Could you check a few things on this drawing? It's one solid part, dimensions in mm from its lowest x, y, z. A direction names the side the tool comes from. Round coordinates to 2 decimals unless told otherwise and drop trailing zeros. Loops run counter-clockwise (first coordinate to the right, second up) from the corner with the lowest first, then second, coordinate; pieces in that order, holes last. Notation, with made-up numbers: M 70.5,62 L 123.5,62 A21 ccw 123.5,91 Z; hole C -6.5,83.5 d1. An arc over 180 degrees is marked long. Put each result on its own line as item: value. Start each with the question number.
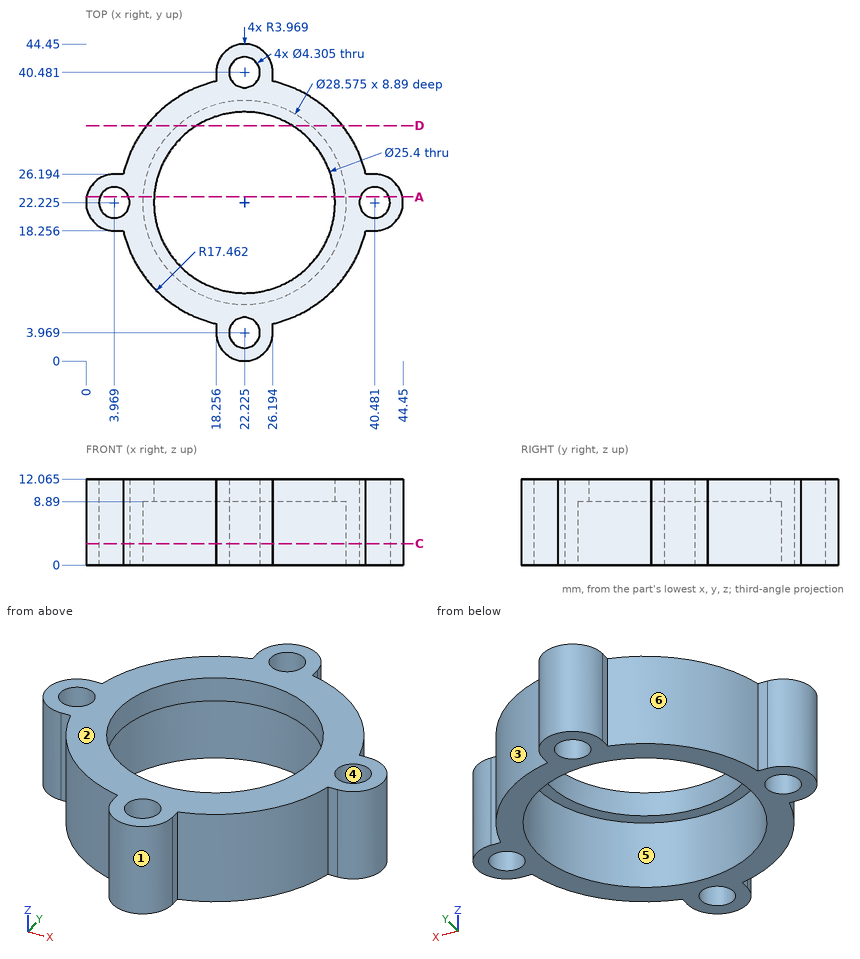
1) If we mould it in two halves opening along Y, with no side actions, what happens to the marked faces 1, 2, 3 and 4? For each: pulls with the +Y half, pulls with the -Y half, needs draft (parallel to the pull), parting line crosses it, or undercut.
2) Suppose I cut it at A-A (y = 23). Write out the boundary of the cut face in (x, z) (1 decimal), plus the area to 3 significant figures.
3) Suppose I cut it at C-C (z = 3). Write out the boundary of the cut face in (x, y) (1 decimal).
4) I'm going to push flat-ended pins straight in: P1, Ø0.6, axis at y = 40, z = 5, coming from the +X side; P2, Ø1, axis at x = 40, z = 8.5, coming from the +Y side; P3, Ø6, axis at y = 12, z = 8, coming from the -X side; P4, Ø8.5, axis at x = 18.5, y = 17.5, coming from the -Z side. Where does each tip first touch, or does it pass through?
5) If I drill on probe 1 along X at (y, z) = (40.5, 10); probe 2 along X at (y, z) = (34, 7) (1 decimal), over which ranges is the centre line in solid material (lowest first)? Write a range as from..to.
6) On a 3-axis mill with a long thin cutter (end or side, diameter ignored), from which of +Z, -Z, +X, -X, +Y, -Y can I reach the whole of each face in a straight line? I mean the marked faces 5 and 6. Say none if no direction works.
7) Suppose I cut it at D-D (y = 33). Write out the boundary of the cut face in (x, z) (1 decimal).
Results are:
1. face 1: pulls with the -Y half
1. face 2: needs draft
1. face 3: pulls with the +Y half
1. face 4: undercut
2. outline: M 0.1,0 L 2,0 L 2,12.1 L 0.1,12.1 Z; M 6,0 L 8,0 L 8,8.9 L 9.5,8.9 L 9.5,12.1 L 6,12.1 Z; M 34.9,8.9 L 36.5,8.9 L 36.5,0 L 38.5,0 L 38.5,12.1 L 34.9,12.1 Z; M 42.5,0 L 44.4,0 L 44.4,12.1 L 42.5,12.1 Z
2. area: 103 mm²
3. outline: M 4,18.3 L 5.2,18.3 A17.5 ccw 18.3,5.2 L 18.3,4 A4 ccw 26.2,4 L 26.2,5.2 A17.5 ccw 39.2,18.3 L 40.5,18.3 A4 ccw 40.5,26.2 L 39.2,26.2 A17.5 ccw 26.2,39.2 L 26.2,40.5 A4 ccw 18.3,40.5 L 18.3,39.2 A17.5 ccw 5.2,26.2 L 4,26.2 A4 ccw Z; hole C 4,22.2 d4.3; hole C 22.2,22.2 d28.6; hole C 22.2,4 d4.3; hole C 22.2,40.5 d4.3; hole C 40.5,22.2 d4.3
4. P1: x = 26.19
4. P2: y = 26.19
4. P3: x = 6.33
4. P4: through
5. probe 1: 18.26..20.07, 24.38..26.19
5. probe 2: 9.3..14.1, 30.3..35.1
6. face 5: -Z
6. face 6: +Z, -Z, -X, +Y
7. outline: M 8.5,0 L 12.8,0 L 12.8,8.9 L 15.5,8.9 L 15.5,12.1 L 8.5,12.1 Z; M 28.9,8.9 L 31.6,8.9 L 31.6,0 L 36,0 L 36,12.1 L 28.9,12.1 Z
